Geometry check sheet. Reference: the model listing, model coordinates, mm. A direction names the side the tool comes from. Give positions to 0.01 mm unless a question says otherwise; leave off trailing zeros. Order: outer loops, then holes, each group sorted by start corner. A loop starts at its lowest first (then second) coordinate and runs counter-clockwise, first axis right, second up. Notation, with made-up numbers: M -2.5,78 L 43.5,78 A13 cw 43.5,87 Z; hole C 32.5,86 d10. An arc over 180 degrees is marked long. Answer as a JSON object with one key per item and string values. Group by question number.
from build123d import *

# Parameters (mm, degrees)
BOSS_EXTRUDE1_DEPTH = 0.285
SKETCH2_W           = 4.9
SKETCH2_H           = 6.35
BOSS_EXTRUDE2_DEPTH = 2
BOSS_EXTRUDE3_DEPTH = 1.555
SKETCH4_W           = 0.635
SKETCH4_H           = 0.635
BOSS_EXTRUDE4_DEPTH = 8.85


with BuildPart() as part:
    # Sketch1 → Boss-Extrude1 (new, symmetric)
    with BuildSketch(Plane(origin=(0, 0, 0), x_dir=(1, 0, 0), z_dir=(0, 1, 0))):
        Polygon((22.1, 3.85), (55.58, 3.85), (56.98, 2.45), (60.9, 2.45), (60.9, -2.45), (56.98, -2.45), (55.58, -3.85), (22.1, -3.85), (22.1, -21.85), (-22.1, -21.85), (-22.1, 21.85), (22.1, 21.85), align=None)
    extrude(amount=BOSS_EXTRUDE1_DEPTH, both=True)

    # Sketch2 → Boss-Extrude2 (add)
    with BuildSketch(Plane(origin=(60.9, 0, 0), x_dir=(0, 0, -1), z_dir=(1, 0, 0))):
        Rectangle(SKETCH2_W, SKETCH2_H)
    extrude(amount=BOSS_EXTRUDE2_DEPTH)

    # Sketch3 → Boss-Extrude3 (add, symmetric)
    with BuildSketch(Plane.XY):
        Polygon((62.9, 3.175), (69.11, 3.175), (69.11, 2.355), (67.63, 1.405), (66.38, 1.405), (64.9, 2.355), (62.9, 2.355), align=None)
    extrude(amount=BOSS_EXTRUDE3_DEPTH, both=True)

    # Sketch4 → Boss-Extrude4 (add)
    with BuildSketch(Plane(origin=(62.9, 0, 0), x_dir=(0, 0, -1), z_dir=(1, 0, 0))):
        with Locations((-1.27, 0)):
            Rectangle(SKETCH4_W, SKETCH4_H)
        with Locations((1.27, 0)):
            Rectangle(SKETCH4_W, SKETCH4_H)
    extrude(amount=BOSS_EXTRUDE4_DEPTH)


solid = part.part
1. Cross-section at B-B (x = -5). Record the cut outline in (y, z) (3 decimals), and give its area (3 significant figures).
2. Depth check by flat-ended pin: pin 1 (0.5 mm diameter, centred on y = 0, z = -14, fed in from +X); pin 2 (0.5 mm diameter, centred on x = 67, y = 2.5, fed in from -Z) (3 decimals); pin 3 (8 mm diameter, centred on x = -9, z = -1.5, fed in from +Y) (3 decimals); pin 4 (1 mm diameter, centred on y = 1.5, z = -3, fed in from -X). Enter the tip coordinate at first touch or a pass-through.
3. Cross-section at C-C (y = -1.5). Record the cut outline in (x, z), and give its area (3 significant figures).
4. Access from +Z, -Z, +X, -X, +Y, -Y to the whole of each face (thin tool, end or side, straight path). Record for faces 1 (the flat face through (2, 0.285, 0)), 2 (the flat face through (2, -0.285, 0)).
5. Cross-section at A-A (z = 0). Record the cut outline in (x, y) (3 decimals).
6. Release check for a two-part mould opening along X. For faces 3 (the flat face through (60.9, 2, 0)), 4 (the flat face through (64, 2.355, 0)), 5 (the flat face through (64, 3.175, 0)) record: released by +X, released by -X, zero draft, split by the parting line, or undercut.
7. Thickness scan on line 1 along Z through (x, y) = (26, 0.25); line 2 along X through (y, z) = (0.25, 10); line 3 along Y through (x, z) = (-18, -12.5) (3 decimals). Record the ranges inside material, lowest first. Write a range as [from, to].
Report:
{
 "1": {"outline": "M -0.285,-21.85 L 0.285,-21.85 L 0.285,21.85 L -0.285,21.85 Z", "area": "24.9 mm2"},
 "2": {"pin 1": "stops at x = 22.1", "pin 2": "stops at z = -1.555", "pin 3": "stops at y = 0.285", "pin 4": "passes through"},
 "3": {"outline": "M 60.9,-2.45 L 62.9,-2.45 L 62.9,2.45 L 60.9,2.45 Z", "area": "9.80 mm2"},
 "4": {"face 1": "+Z, -Z, -X, +Y", "face 2": "+Z, -Z, -X, -Y"},
 "5": {"outline": "M -22.1,-0.285 L 60.9,-0.285 L 60.9,-3.175 L 62.9,-3.175 L 62.9,2.355 L 64.9,2.355 L 66.38,1.405 L 67.63,1.405 L 69.11,2.355 L 69.11,3.175 L 60.9,3.175 L 60.9,0.285 L -22.1,0.285 Z"},
 "6": {"face 3": "released by -X", "face 4": "undercut", "face 5": "zero draft"},
 "7": {"line 1": "z = [-3.85, 3.85]", "line 2": "x = [-22.1, 22.1]", "line 3": "y = [-0.285, 0.285]"}
}
